Geometry check sheet. Reference: the model listing, model coordinates, mm. Face numbers are marked on the shaded views. A direction names the side the tool comes from. Round coordinates to 2 decimals unless told otherwise and drop trailing zeros. Order: outer loops, then holes, each group sorted by start corner. A loop starts at its lowest first (then second) coordinate and runs counter-clockwise, first axis right, second up.
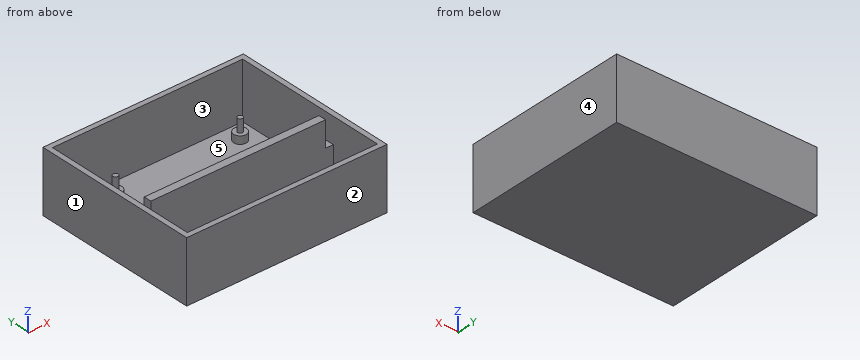
```python
from build123d import *

# Parameters (mm, degrees)
SKETCH1_W           = 78
SKETCH1_H           = 65
BOSS_EXTRUDE1_DEPTH = 24
SKETCH2_W           = 74
SKETCH2_H           = 61
CUT_EXTRUDE1_DEPTH  = 22
SKETCH3_W           = 74
SKETCH3_H           = 3
BOSS_EXTRUDE2_DEPTH = 22
SKETCH4_W           = 3
SKETCH4_H           = 3
CUT_EXTRUDE2_DEPTH  = 10
SKETCH5_R           = 2.5
BOSS_EXTRUDE3_DEPTH = 3
SKETCH6_R           = 1
BOSS_EXTRUDE4_DEPTH = 5


with BuildPart() as part:
    # Sketch1 → Boss-Extrude1 (new body)
    with BuildSketch(Plane.XY):
        with Locations((39, 32.5)):
            Rectangle(SKETCH1_W, SKETCH1_H)
    extrude(amount=BOSS_EXTRUDE1_DEPTH)

    # Sketch2 → Cut-Extrude1 (cut)
    with BuildSketch(Plane.XY.offset(24)):
        with Locations((39, 32.5)):
            Rectangle(SKETCH2_W, SKETCH2_H)
    extrude(amount=-CUT_EXTRUDE1_DEPTH, mode=Mode.SUBTRACT)

    # Sketch3 → Boss-Extrude2 (add)
    with BuildSketch(Plane.XY.offset(2)):
        with Locations((39, 23.5)):
            Rectangle(SKETCH3_W, SKETCH3_H)
    extrude(amount=BOSS_EXTRUDE2_DEPTH)

    # Sketch4 → Cut-Extrude2 (cut)
    with BuildSketch(Plane.XY.offset(24)):
        with Locations((3.5, 23.5)):
            Rectangle(SKETCH4_W, SKETCH4_H)
        with Locations((74.5, 23.5)):
            Rectangle(SKETCH4_W, SKETCH4_H)
    extrude(amount=-CUT_EXTRUDE2_DEPTH, mode=Mode.SUBTRACT)

    # Sketch5 → Boss-Extrude3 (add)
    with BuildSketch(Plane.XY.offset(2)):
        with Locations((20.5, 56)):
            Circle(SKETCH5_R)
        with Locations((69, 56)):
            Circle(SKETCH5_R)
    extrude(amount=BOSS_EXTRUDE3_DEPTH)

    # Sketch6 → Boss-Extrude4 (add)
    with BuildSketch(Plane.XY.offset(5)):
        with Locations((20.5, 56)):
            Circle(SKETCH6_R)
        with Locations((69, 56)):
            Circle(SKETCH6_R)
    extrude(amount=BOSS_EXTRUDE4_DEPTH)


solid = part.part
```
(1) Sectioned sample at C-C, the plane x = 57.5. Record the cut outline in (y, z).
Returned:
outline: (0, 0) - (65, 0) - (65, 24) - (63, 24) - (63, 2) - (25, 2) - (25, 24) - (22, 24) - (22, 2) - (2, 2) - (2, 24) - (0, 24) - close
(2) Draft check along Y on the marked faces 1, 2 and 3. Enter one of: released by +Y, released by -Y, zero draft, split by the parting line, or undercut.
Returned:
face 1: zero draft
face 2: released by -Y
face 3: undercut
(3) Set-up check for the marked faces 4 and 5: record each of +Z, -Z, +X, -X, +Y, -Y from which the full face is reachable in a straight line by a thin tool's end or side.
Returned:
face 4: +Z, -Z, +X, +Y, -Y
face 5: +Z
(4) Depth check by flat-ended pin: P1, Ø4, axis at x = 68, y = 56, coming from the +Z side. Enter the tip coordinate at first touch or a pass-through.
Returned:
P1: stops at z = 10
(5) Sectioned sample at A-A, the plane z = 19. Record the cut outline in (x, y), and give its area (3 significant figures).
Returned:
outline: (0, 0) - (78, 0) - (78, 65) - (0, 65) - close; (5, 22) - (73, 22) - (73, 25) - (5, 25) - close; hole (2, 2) - (76, 2) - (76, 63) - (2, 63) - close
area: 760 mm2
(6) Material ranges on line 1 (Y direction, x = 8, z = 12); line 2 (X direction, y = 3, z = 10.25); line 3 (Y direction, x = 74, z = 22.5), recorded low to high.
Returned:
line 1: y = 0 to 2, 22 to 25, 63 to 65
line 2: x = 0 to 2, 76 to 78
line 3: y = 0 to 2, 63 to 65
(7) Sectioned sample at B-B, the plane z = 7.25. Record the cut outline in (x, y), and give its area (3 significant figures).
Returned:
outline: (0, 0) - (78, 0) - (78, 65) - (0, 65) - close; circle Ø2 at (20.5, 56); circle Ø2 at (69, 56); hole (2, 2) - (76, 2) - (76, 22) - (2, 22) - close; hole (2, 25) - (76, 25) - (76, 63) - (2, 63) - close
area: 784 mm2
(8) Sectioned sample at D-D, the plane y = 15.5. Record the cut outline in (x, z).
Returned:
outline: (0, 0) - (78, 0) - (78, 24) - (76, 24) - (76, 2) - (2, 2) - (2, 24) - (0, 24) - close
